The listing builds one solid part. Answer for the finished solid, in the listing's coordinates (mm). Round coordinates to 2 decimals unless told otherwise and drop trailing zeros. Loops run counter-clockwise (first coordinate to the right, second up) from the corner with the lowest first, then second, coordinate; pieces in that order, holes last. Notation, with made-up numbers: (-4.75, -31.75) - (54.25, -31.75) arc R26 ccw to (54.25, 2.25) - close; hole circle Ø10 at (-29.75, -10). An arc over 180 degrees is marked (long way). One line per item, written item: value.
```python
from build123d import *

# Parameters (mm, degrees)
ESBO_O1_W                = 20.5
ESBO_O1_H                = 21
RESSALTO_EXTRUS_O1_DEPTH = 0.8
ESBO_O2_R                = 0.5
ESBO_O2_R_2              = 1.2
ESBO_O2_R_3              = 0.45
ESBO_O2_R_4              = 0.478821701
CORTE_EXTRUS_O1_DEPTH    = 5


with BuildPart() as part:
    # Esboço1 → Ressalto-extrusão1 (new body)
    with BuildSketch(Plane(origin=(0, 0, 0), x_dir=(1, 0, 0), z_dir=(0, 1, 0))):
        Rectangle(ESBO_O1_W, ESBO_O1_H)
    extrude(amount=RESSALTO_EXTRUS_O1_DEPTH)

    # Esboço2 → Corte-extrusão1 (cut, symmetric)
    with BuildSketch(Plane(origin=(0, 0.8, 0), x_dir=(1, 0, 0), z_dir=(0, 1, 0))):
        with Locations(Location((8.169588965, 9.121369329, 0), (0, 0, 90))):
            Circle(ESBO_O2_R)
        with Locations(Location((8.656271278, 1.430267657, 0), (0, 0, 90))):
            Circle(ESBO_O2_R)
        with Locations(Location((8.656271278, -4.425515861, 0), (0, 0, 90))):
            Circle(ESBO_O2_R)
        with Locations(Location((8.656271278, -6.946579519, 0), (0, 0, 90))):
            Circle(ESBO_O2_R)
        with Locations(Location((6.475637733, -3.207774386, 0), (0, 0, 90))):
            Circle(ESBO_O2_R_2)
        with Locations(Location((-6.84447605, -3.207774386, 0), (0, 0, 90))):
            Circle(ESBO_O2_R_2)
        with Locations(Location((-8.701687341, -5.133968427, 0), (0, 0, 90))):
            Circle(ESBO_O2_R)
        with Locations(Location((-8.701687341, -7.706335777, 0), (0, 0, 90))):
            Circle(ESBO_O2_R)
        with Locations(Location((4.836575481, 9.121369329, 0), (0, 0, 90))):
            Circle(ESBO_O2_R_3)
        with Locations(Location((2.76166475, 9.121369329, 0), (0, 0, 90))):
            Circle(ESBO_O2_R_3)
        with Locations(Location((1.691416538, 6.593096738, 0), (0, 0, 90))):
            Circle(ESBO_O2_R)
        with Locations(Location((-8.994083212, 0.392498409, 0), (0, 0, 90))):
            Circle(ESBO_O2_R)
        with Locations(Location((-3.86010674, -0.657838238, 0), (0, 0, 90))):
            Circle(ESBO_O2_R)
        with Locations(Location((-1.120283175, -0.657838238, 0), (0, 0, 90))):
            Circle(ESBO_O2_R)
        with Locations(Location((0.809655437, -0.657838238, 0), (0, 0, 90))):
            Circle(ESBO_O2_R)
        with Locations(Location((3.446089433, -0.657838238, 0), (0, 0, 90))):
            Circle(ESBO_O2_R)
        with Locations(Location((1.691416538, 4.045324666, 0), (0, 0, 90))):
            Circle(ESBO_O2_R)
        with Locations(Location((-6.451906001, 8.700562352, 0), (0, 0, 90))):
            Circle(ESBO_O2_R_4)
        with Locations(Location((-6.038262859, 6.619037193, 0), (0, 0, 90))):
            Circle(ESBO_O2_R_4)
        with Locations(Location((-8.92956931, 7.368379214, 0), (0, 0, 90))):
            Circle(ESBO_O2_R_4)
        with Locations(Location((-6.038262859, 4.017675665, 0), (0, 0, 90))):
            Circle(ESBO_O2_R)
        with Locations(Location((-7.392078127, 2.439818031, 0), (0, 0, 90))):
            Circle(ESBO_O2_R)
    extrude(amount=CORTE_EXTRUS_O1_DEPTH, both=True, mode=Mode.SUBTRACT)


solid = part.part
```
1) A cutting plane is placed at B-B on z = -0.25. Give the vertices of the cut face in (x, y), and give its area (3 significant figures).
Final values:
outline: (-10.25, 0) - (-9.47, 0) - (-9.47, 0.8) - (-10.25, 0.8) - close; (-8.51, 0) - (10.25, 0) - (10.25, 0.8) - (-8.51, 0.8) - close
area: 15.6 mm2
2) For a pull along Z with two mould halves and no side action, classify faces 1 (the flat face through (0, 0.8, 0)), 2 (the cylindrical face through (-9.49, 0.41, -0.33)) as released by +Z, released by -Z, zero draft, split by the parting line, or undercut.
Final values:
face 1: zero draft
face 2: undercut
3) Consider L1, parallel to X at y = 0.4, z = 3.25; L2, parallel to X at y = 0.5, z = 3.5; L3, parallel to X at y = 0.5, z = 0.5. Determine where each line is inside the solid, lowest interval first.
Final values:
L1: -10.25 to -8.04, -5.65 to 5.28, 7.67 to 10.25
L2: -10.25 to -8.01, -5.68 to 5.31, 7.64 to 10.25
L3: -10.25 to -4.33, -3.39 to -1.59, -0.65 to 0.34, 1.28 to 2.97, 3.92 to 10.25
4) A cutting plane is placed at A-A on y = 0.65. Give the number of separate pieces and of enclosed holes in the cut face, and give its area (3 significant figures).
Final values:
separate pieces: 1
enclosed holes: 22
area: 406 mm2
5) This flat-tipped pin is pushed along its axis until it touches: pin 1 Ø3 at (x, z) = (-6.84, 3.21) entering from -Y. Where does it stop, or does it pass through?
Final values:
pin 1: y = 0
